Part model, mm, in its own coordinate system. A direction names the side the tool comes from. Coordinates: 2 decimals unless noted, no trailing zeros. Loops run counter-clockwise (first coordinate to the right, second up) from the corner with the lowest first, then second, coordinate; pieces in that order, holes last. Notation, with made-up numbers: M 26.25,5 L 30.25,5 A35 cw 30.25,42 Z; hole C 43,82.5 d3. An arc over 180 degrees is marked long. Answer as CSV lines item,"result". Start each with the question number.
from build123d import *

# Parameters (mm, degrees)
EXTRUDE004_DEPTH = 5
EXTRUDE003_DEPTH = 10
FILLET021_R      = 1


with BuildPart() as extrude004:
    # Sketch006 → Extrude004 (new body)
    with BuildSketch(Plane.XZ):
        with BuildLine():
            ThreePointArc((14.771842, 0.154152), (17.827348, 3.62591), (14.461083, 6.797264))
            Line((14.461083, 6.797264), (12.252875, 6.797264))
            Line((12.252875, -5.267611), (12.252875, 6.797264))
            Line((5.422805, -5.82309), (12.252875, -5.267611))
            ThreePointArc((5.422805, -5.82309), (2.802341, -9.576998), (6.556249, -12.197462))
            Line((6.556249, -12.197462), (14.771842, -12.197462))
            Line((14.771842, -12.197462), (14.771842, 0.154152))
        make_face()
    extrude(amount=EXTRUDE004_DEPTH)


with BuildPart() as extrude004_1:
    # Extrude004 placement: moved
    add(extrude004.part.moved(Location((0, -8, 0))))


with BuildPart() as fillet021:
    # Sketch005 → Extrude003 (new body)
    with BuildSketch(Plane.XY):
        Polygon((57.709053, -19.346786), (57.709053, -22.346786), (65.709053, -22.346786), (65.709053, -10.346786), (62.709053, -10.346786), (62.709053, -19.346786), align=None)
    extrude(amount=EXTRUDE003_DEPTH)


with BuildPart() as fillet021_1:
    # Extrude003 placement: moved
    add(fillet021.part.moved(Location((0, 0, -14))))

    # Fillet021
    fillet021_edges = [fillet021_1.edges().sort_by_distance(p)[0] for p in [
        (57.709053, -19.346786, -9),
        (57.709053, -22.346786, -9),
        (65.709053, -22.346786, -9),
        (61.709053, -22.346786, -4),
        (65.709053, -10.346786, -9),
        (65.709053, -16.346786, -4),
        (62.709053, -10.346786, -9),
        (64.209053, -10.346786, -4),
        (62.709053, -19.346786, -9),
        (62.709053, -14.846786, -4),
        (60.209053, -19.346786, -4),
    ]]
    fillet(fillet021_edges, radius=FILLET021_R)


with BuildPart() as fillet021_2:
    # Fillet021 placement: moved
    add(fillet021_1.part.moved(Location((0, 0, 0.4))))


with BuildPart() as c4holds002:
    # Part__Mirroring005: instance of Fillet021
    add(fillet021_2.part.mirror(Plane(origin=(0, 0, 0), x_dir=(0, -1, 0), z_dir=(1, 0, 0))))


with BuildPart() as c4holds002_1:
    # Part__Mirroring005 placement: moved
    add(c4holds002.part.moved(Location((78, 0, 0.4))))

    # Fusion040: union Extrude004
    add(extrude004_1.part)


solid = c4holds002_1.part
Q1. Two-plate mould, pull along Z, no slides. Class faces 1 (the face through (14, -19, -3.2)), 2 (the face through (15.006, -14.896, -3.501)), 3 (the face through (12.576, -10.647, -12.692)): +Z half, -Z half, draft (parallel to the pull), parting line (faces both ways), or undercut.
Q2. Tool access for faces 4 (the face through (18, -19.347, -9)), 5 (the face through (12.253, -10, 1)), 6 (the face through (12.576, -17.115, -3.501)): list every direction of +Z, -Z, +X, -X, +Y, -Y with a clear straight run to the whole face (end or side of a thin tool).
Q3. Wall check: L1, parallel to Y at x = 15.25, z = 5; L2, parallel to X at y = -11.5, z = -5; L3, parallel to X at y = -10.75, z = 3.5. Give the ranges that are in metal, low to high.
Q4. Slice it at B-B, the plane y = -12.5. Write the cut outline in (x, z), and give its area (3 significant figures).
Q5. Slice it at D-D, the plane x = 17. Write the cut outline in (y, z).
Q6. Flat gauge pins, fed straight in: P1, Ø2.5, axis at x = 18, z = -7.5, coming from the +Y side; P2, Ø4.5, axis at x = 13, z = -0.5, coming from the -Y side; P3, Ø3, axis at y = -9.5, z = -3, coming from the +X side. Where does each tip first touch, or does it go through?
Q7. Slice it at C-C, the plane x = 14. Write the cut outline in (y, z).
Solved:
1,face 1,"+Z half"
1,face 2,"undercut"
1,face 3,"draft"
2,face 4,"+Z, -Z, +X, +Y"
2,face 5,"+Z, -X, +Y, -Y"
2,face 6,"+Z, -X, -Y"
3,L1,"y = -13 to -8"
3,L2,"x = 12.25 to 15.29"
3,L3,"x = 12.25 to 17.83"
4,outline,"M 5.42,-5.82 A3.24 ccw 6.56,-12.2 L 12.29,-12.2 L 12.29,-13.2 L 15.29,-13.2 L 15.29,-4.2 A1 ccw 14.77,-3.32 L 14.77,0.15 A3.33 ccw 14.46,6.8 L 12.25,6.8 L 12.25,-5.27 Z"
4,area,"129 mm2"
5,outline,"M -22.35,-13.2 L -19.35,-13.2 L -19.35,-4.2 A1 ccw -20.35,-3.2 L -21.35,-3.2 A1 ccw -22.35,-4.2 Z; M -13,1.27 L -8,1.27 L -8,5.67 L -13,5.67 Z"
6,P1,"stops at y = -19.35"
6,P2,"stops at y = -13"
6,P3,"stops at x = 15"
7,outline,"M -22.35,-13.2 L -10.35,-13.2 L -10.35,-12.2 L -8,-12.2 L -8,6.8 L -13,6.8 L -13,-3.2 L -21.35,-3.2 A1 ccw -22.35,-4.2 Z"
